from build123d import *

# Parameters (mm, degrees)
F2_DEPTH = 12.5
F4_DEPTH = 50
F6_D     = 5
F6_DEPTH = 50
F6_TIP   = 1.5021515476
F7_W     = 8.875
F7_H     = 21.375
F8_DEPTH = 5
F9_R     = 3.625
F10_R    = 4


# Not quite as in the source:
# - a feature names something its author has since deleted; it is built from what else it names


with BuildPart() as f1:
    # F0 (on Right) → F1 (revolve)
    with BuildSketch(Plane.YZ):
        Polygon((-25, 22.5), (-100, 22.5), (-100, 20), (0, 20), (100, 20), (160, 20), (160, 22.5), (100, 22.5), (25, 22.5), (0, 22.5), align=None)
    revolve(axis=Axis((0, 2.0652181371, 0), (0, 1, 0)))

    # F0 (on Right) → F2 (join, symmetric)
    with BuildSketch(Plane.YZ):
        Polygon((-25, 42.5), (-25, 22.5), (0, 22.5), (25, 22.5), (25, 42.5), (0, 42.5), align=None)
    extrude(amount=F2_DEPTH, both=True)

    # F3 (on face) → F4 (join)
    with BuildSketch(Plane(origin=(0, 25, 0), x_dir=(-1, 0, 0), z_dir=(0, 1, 0))):
        Polygon((0, 22.5), (-12.5, 22.5), (-12.5, 18.6568256468), align=None)
        Polygon((12.5, 22.5), (0, 22.5), (12.5, 18.6568256468), align=None)
    extrude(amount=-F4_DEPTH)

    # F6
    with Locations(Plane.XY.offset(42.5)):
        with Locations((0, 0)):
            Hole(F6_D / 2, depth=F6_DEPTH)
            with Locations((0, 0, -(F6_DEPTH + F6_TIP / 2))):  # 118° drill point
                Cone(0, F6_D / 2, F6_TIP, mode=Mode.SUBTRACT)

    # F7 (on face) → F8 (join)
    with BuildSketch(Plane.XY.offset(42.5)):
        with Locations((-8.0625, -14.3125)):
            Rectangle(F7_W, F7_H)
    extrude(amount=F8_DEPTH)

    # F9
    f9_edges = [f1.edges().sort_by_distance(p)[0] for p in [
        (-3.625, -3.625, 45),
    ]]
    fillet(f9_edges, radius=F9_R)

    # F10
    f10_edges = [f1.edges().sort_by_distance(p)[0] for p in [
        (12.5, 25, 30.604143),
        (12.5, -25, 30.604143),
        (-12.5, 25, 30.604143),
        (-12.5, -25, 33.104143),
    ]]
    fillet(f10_edges, radius=F10_R)


solid = f1.part
Can you work these out from the model? Positions are in its coordinate system, mm. A direction names the side the tool comes from. Coordinates: 2 decimals unless noted, no trailing zeros. Loops run counter-clockwise (first coordinate to the right, second up) from the corner with the lowest first, then second, coordinate; pieces in that order, holes last. Notation, with made-up numbers: (29, 19) - (86, 19) arc R17 cw to (86, 42) - close; hole circle Ø11 at (-9, 9.5). An arc over 180 degrees is marked (long way). Put each result on its own line as item: value. Start each with the question number.
Item 1: For pin 1 (4 mm diameter, centred on y = 102.5, z = 6, fed in from +X); pin 2 (8 mm diameter, centred on x = 0, y = 0, fed in from +Z); pin 3 (4 mm diameter, centred on y = 129, z = 8.5, fed in from -X), each with a flat end and sliding along its axis, tell me the tip position at first contact or that it passes through.
Item 2: If I drill on line 1 along X through (y, z) = (100, 0); line 2 along X through (y, z) = (0, 32.25); line 3 along Y through (x, z) = (0, 29), over which ranges is the centre line in solid material (lowest first)?
Item 3: Suppose I cut it at B-B (y = 0). Please give me the cut outline in (x, z), and give its area (3 significant figures).
Item 4: Which directions (+Z, -Z, +X, -X, +Y, -Y) give clear straight access to the entire face, cutting with the end or side of a thin tool? Please do faces 1 (the face through (3, 0, 42.5)), 2 (the face through (-19.524, 31.82, -4.336)), 3 (the face through (-1.6, -100, -20.1)), 4 (the face through (12.5, 0, 31)), 5 (the face through (-10, -3.625, 45)).
Item 5: Suppose I cut it at C-C (x = 0). Please give me the cut outline in (y, z).
Item 6: Suppose I cut it at D-D (z = 39). Please give me the cut outline in (x, y).
Item 7: If we mould it in two halves opening along Y, with no side actions, what happens to faces 6 (the face through (0, -25, 34)), 7 (the face through (0.54, -2.44, 31.01)), 8 (the face through (-1.6, 160, 20.1)), 9 (the face through (-12.5, 0, 33))? For each: +Y half, -Y half, draft (parallel to the pull), parting line (faces both ways), or undercut.
Item 8: Suppose I cut it at A-A (z = 0). Please give me the cut outline in (x, y).
Here are the results:
1. pin 1: x = 22.14
1. pin 2: z = 42.5
1. pin 3: x = -21.54
2. line 1: -22.5 to -20, 20 to 22.5
2. line 2: -12.5 to -2.5, 2.5 to 12.5
2. line 3: -25 to -2.5, 2.5 to 25
3. outline: (-12.5, 18.71) arc R22.5 ccw (long way) to (12.5, 18.71) - (12.5, 42.5) - (2.5, 42.5) - (2.5, 19.84) arc R20 cw (long way) to (-2.5, 19.84) - (-2.5, 42.5) - (-12.5, 42.5) - close
3. area: 751 mm²
4. face 1: +Z, +X, +Y
4. face 2: +Y, -Y
4. face 3: +Z, -Z, +X, -X, -Y
4. face 4: +Z, +X, +Y, -Y
4. face 5: +Z, +X, -X, +Y
5. outline: (-100, -22.5) - (160, -22.5) - (160, -20) - (-100, -20) - close; (-100, 20) - (-2.5, 20) - (-2.5, 42.5) - (-25, 42.5) - (-25, 22.5) - (-100, 22.5) - close; (2.5, 20) - (160, 20) - (160, 22.5) - (25, 22.5) - (25, 42.5) - (2.5, 42.5) - close
6. outline: (-12.5, -21) arc R4 ccw to (-8.5, -25) - (8.5, -25) arc R4 ccw to (12.5, -21) - (12.5, 21) arc R4 ccw to (8.5, 25) - (-8.5, 25) arc R4 ccw to (-12.5, 21) - close; hole circle Ø5 at (0, 0)
7. face 6: -Y half
7. face 7: undercut
7. face 8: +Y half
7. face 9: draft
8. outline: (-22.5, -100) - (-20, -100) - (-20, 160) - (-22.5, 160) - close; (20, -100) - (22.5, -100) - (22.5, 160) - (20, 160) - close
